from build123d import *

# Parameters (mm, degrees)
F0_W      = 144.78
F0_H      = 81.28
F1_DEPTH  = 45.72
F2_W      = 104.14
F2_H      = 81.28
F3_DEPTH  = 13.97
F4_W      = 20.32
F4_H      = 40.64
F5_DEPTH  = 24.13
F6_W      = 72.39
F6_H      = 81.28
F7_DEPTH  = 12.7
F8_R      = 12.7
F9_DEPTH  = 32.004
F10_R     = 12.7
F11_DEPTH = 19.558


with BuildPart() as f1:
    # F0 (on Top) → F1 (new body)
    with BuildSketch(Plane.XY):
        with Locations((1.572737, 9.473312)):
            Rectangle(F0_W, F0_H)
    extrude(amount=F1_DEPTH)

    # F2 (on face) → F3 (cut)
    with BuildSketch(Plane.XY.offset(45.72)):
        with Locations((1.572737, 9.473312)):
            Rectangle(F2_W, F2_H)
    extrude(amount=-F3_DEPTH, mode=Mode.SUBTRACT)

    # F4 (on face) → F5 (cut)
    with BuildSketch(Plane.XY.offset(45.72)):
        with Locations((63.802737, 9.473312)):
            Rectangle(F4_W, F4_H)
    extrude(amount=-F5_DEPTH, mode=Mode.SUBTRACT)

    # F6 (on face) → F7 (cut)
    with BuildSketch(Plane(origin=(0, 0, 0), x_dir=(1, 0, 0), z_dir=(0, 0, -1))):
        with Locations((37.767737, -9.473312)):
            Rectangle(F6_W, F6_H)
    extrude(amount=-F7_DEPTH, mode=Mode.SUBTRACT)

    # F8 (on face) → F9 (cut)
    with BuildSketch(Plane.XY.offset(31.75)):
        with Locations((-25.097263, 9.473312)):
            Circle(F8_R)
    extrude(amount=-F9_DEPTH, mode=Mode.SUBTRACT)

    # F10 (on face) → F11 (cut)
    with BuildSketch(Plane.XY.offset(31.75)):
        with Locations((26.972737, 9.473312)):
            Circle(F10_R)
    extrude(amount=-F11_DEPTH, mode=Mode.SUBTRACT)


solid = f1.part
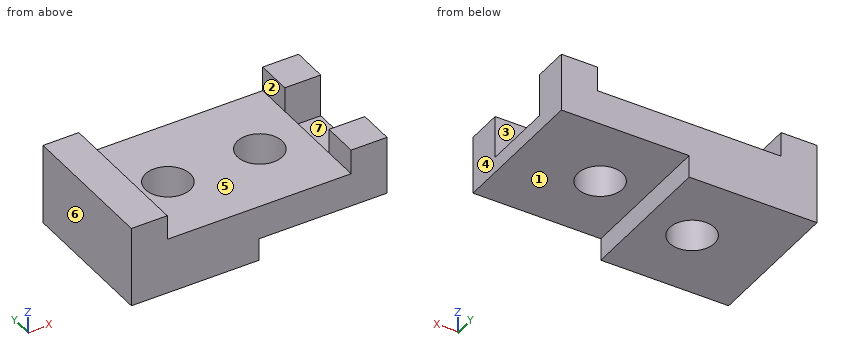
Part model, mm, in its own coordinate system. Face numbers are marked on the shaded views. A direction names the side the tool comes from. Coordinates: 2 decimals unless noted, no trailing zeros. Order: outer loops, then holes, each group sorted by start corner. A loop starts at its lowest first (then second) coordinate and runs counter-clockwise, first axis right, second up. Notation, with made-up numbers: (5, 51.25) - (56, 51.25) arc R24 ccw to (56, 69.25) - close; hole circle Ø5 at (56.5, 10). An arc over 180 degrees is marked (long way). Use CSV: the item, a comma, the result in double quotes.
Item 1: Probe probe 1 along X at (y, z) = (9.5, 29); probe 2 along X at (y, z) = (-21, 41); probe 3 along Y at (x, z) = (63, 24). List the from-to ranges inside material, lowest first.
Solved:
probe 1,"x = -70.82 to -37.8, -12.4 to 14.27, 39.67 to 53.64"
probe 2,"x = -70.82 to -50.5, 53.64 to 73.96"
probe 3,"y = -31.17 to -10.85, 29.79 to 50.11"
Item 2: Mould opens along X. For the marked faces 4, 5, 6 and 7 say: +X half, -X half, draft (parallel to the pull), parting line (faces both ways), or undercut.
Solved:
face 4,"+X half"
face 5,"undercut"
face 6,"-X half"
face 7,"draft"
Item 3: Saw through at C-C on y = -19. Give the cut face in (x, z).
Solved:
outline,"(-70.82, 0) - (1.57, 0) - (1.57, 12.7) - (73.96, 12.7) - (73.96, 45.72) - (53.64, 45.72) - (53.64, 31.75) - (-50.5, 31.75) - (-50.5, 45.72) - (-70.82, 45.72) - close"
Item 4: 3-axis set-ups, long thin cutter, end or side, ignore diameter. For the marked faces 1, 2 and 3: which of +Z, -Z, +X, -X, +Y, -Y reach the whole face in a straight line?
Solved:
face 1,"-Z, +X, +Y, -Y"
face 2,"+Z, +Y, -Y"
face 3,"+Z, +X"
Item 5: Saw through at B-B on x = -15. Give the cut face in (y, z), and give its area (3 significant figures).
Solved:
outline,"(-31.17, 0) - (1.77, 0) - (1.77, 31.75) - (-31.17, 31.75) - close; (17.18, 0) - (50.11, 0) - (50.11, 31.75) - (17.18, 31.75) - close"
area,"2,090 mm²"
Item 6: Drop flat-ended pins along their axis: P1, Ø1.5, axis at y = 23, z = 28.5, coming from the +X side; P2, Ø4, axis at y = 4, z = 36.5, coming from the +X side; P3, Ø6, axis at x = 68, y = 8, coming from the +Z side. Give the stop position or say it passes through.
Solved:
P1,"stops at x = 53.64"
P2,"stops at x = -50.5"
P3,"stops at z = 21.59"
Item 7: Saw through at D-D on y = 18.5. Give the cut face in (x, z), and give its area (3 significant figures).
Solved:
outline,"(-70.82, 0) - (-34.03, 0) - (-34.03, 31.75) - (-50.5, 31.75) - (-50.5, 45.72) - (-70.82, 45.72) - close; (-16.16, 0) - (1.57, 0) - (1.57, 12.7) - (18.04, 12.7) - (18.04, 31.75) - (-16.16, 31.75) - close; (35.91, 12.7) - (73.96, 12.7) - (73.96, 21.59) - (53.64, 21.59) - (53.64, 31.75) - (35.91, 31.75) - close"
area,"2,850 mm²"
Item 8: Saw through at A-A on z = 36. Give the cut face in (x, y).
Solved:
outline,"(-70.82, -31.17) - (-50.5, -31.17) - (-50.5, 50.11) - (-70.82, 50.11) - close; (53.64, -31.17) - (73.96, -31.17) - (73.96, -10.85) - (53.64, -10.85) - close; (53.64, 29.79) - (73.96, 29.79) - (73.96, 50.11) - (53.64, 50.11) - close"
